from build123d import *

# Parameters (mm, degrees)
SKETCH1_W           = 16.5
SKETCH1_H           = 15.5
SKETCH1_W_2         = 12.5
SKETCH1_H_2         = 11.742424242
BOSS_EXTRUDE1_DEPTH = 5
BOSS_EXTRUDE2_DEPTH = 10
CUT_SWEEP1_START    = -6
CUT_SWEEP1_DEPTH    = 12


# Read off the part's stored shape, not the designer's step: Cut-Sweep1
with BuildPart() as part:
    # Sketch1 → Boss-Extrude1 (new body)
    with BuildSketch(Plane.XY):
        Rectangle(SKETCH1_W, SKETCH1_H)
        Rectangle(SKETCH1_W_2, SKETCH1_H_2, mode=Mode.SUBTRACT)
    extrude(amount=BOSS_EXTRUDE1_DEPTH)

    # Sketch3 → Boss-Extrude2 (add, symmetric)
    with BuildSketch(Plane(origin=(0, 0, 0), x_dir=(0, 0, -1), z_dir=(1, 0, 0))):
        with BuildLine():
            Line((13.022755533, 1.177389365), (0, -9.75))
            Line((0, -9.75), (0, 9.75))
            ThreePointArc((0, 9.75), (7.794535943, 7.412955642), (13.022755533, 1.177389365))
        make_face()
    extrude(amount=BOSS_EXTRUDE2_DEPTH, both=True)

    # Cut-Sweep1 outline → Cut-Sweep1 (cut)
    with BuildSketch(Plane.YZ.offset(CUT_SWEEP1_START)):
        Polygon((-3.793172037, -7.099071125), (4.667171481, 0), (-4.667171481, 0), (-7.649897695, -2.502804467), align=None)
    extrude(amount=CUT_SWEEP1_DEPTH, mode=Mode.SUBTRACT)


solid = part.part
Geometry: final body of the model. Coordinates: model frame, mm. A direction names the side the tool comes from. Give positions to 0.01 mm unless a question says otherwise; leave off trailing zeros. Write each loop counter-clockwise with the first axis right and the second up, starting at its lowest first coordinate (ties: lowest second). Pieces come first, ordered by that corner, then holes. Notation, with made-up numbers: M -40,6 L -23,6 A5 ccw -23,10 Z; hole C -8.75,-31 d1. An arc over 180 degrees is marked long. Answer in a Markdown table with one row per item. Add a question column.
(1) Section A-A on z = 0.5. Return loops of the section in (x, y), and give its area (3 significant figures).
(2) Section D-D on y = -7.25. Return loops of the section in (x, z), and give its area (3 significant figures).
(3) Ray query, line 1 (X direction, y = -3.5, z = 1.75); line 2 (X direction, y = -1.5, z = -1); line 3 (Y direction, x = -7.25, z = 1.75). Return the intervals inside material, ascending.
(4) Section C-C on x = -7.25. Return loops of the section in (y, z), and give its area (3 significant figures).
(5) First-contact query: pin 1 (2.5 mm diameter, centred on y = -2, z = 2, fed in from +X); pin 2 (1 mm diameter, centred on x = 6.5, z = -4.5, fed in from +Y); pin 3 (10 mm diameter, centred on x = 4, z = -4, fed in from +Y); pin 4 (2.5 mm diameter, centred on x = 1.5, z = 2.5, fed in from -Y). Flat tips, straight axial feed; report the tip coordinate or a pass-through.
(6) Mould query, pull axis Y, two halves, no side actions, for faces 6 (the flat face through (0, -5.871, 2)), 7 (the flat face through (0, -7, 5)), 8 (the flat face through (0, -7.75, 2)). Classes: +Y half, -Y half, draft (parallel to the pull), parting line (faces both ways), or undercut.
(7) Reachability of faces 1 (the flat face through (-0.1, -6.1, -1.2)), 2 (the flat face through (1, -5, 0)), 3 (the flat face through (-8.25, 0, 2)), 4 (the flat face through (0, 7.75, 2)), 5 (the flat face through (-6, -2, -3)) from +Z, -Z, +X, -X, +Y, -Y: full face, straight path, thin tool, end or side. Return the list, or none.
(8) Section B-B on x = 0.75. Return loops of the section in (y, z).
Result set:
| question | item | result |
|---|---|---|
| 1 | outline | M -8.25,-7.75 L 8.25,-7.75 L 8.25,7.75 L -8.25,7.75 Z; hole M -6.25,-5.87 L 6.25,-5.87 L 6.25,5.87 L -6.25,5.87 Z |
| 1 | area | 109 mm^2 |
| 2 | outline | M -10,-2.98 L -6,-2.98 L -6,-2.17 L 6,-2.17 L 6,-2.98 L 10,-2.98 L 10,0 L 8.25,0 L 8.25,5 L -8.25,5 L -8.25,0 L -10,0 Z |
| 2 | area | 132 mm^2 |
| 3 | line 1 | x = -8.25 to -6.25, 6.25 to 8.25 |
| 3 | line 2 | x = -10 to -6, 6 to 10 |
| 3 | line 3 | y = -7.75 to 7.75 |
| 4 | outline | M -9.75,0 L 1.18,-13.02 A14.19 ccw 9.75,0 L 7.75,0 L 7.75,5 L -7.75,5 L -7.75,0 Z |
| 4 | area | 229 mm^2 |
| 5 | pin 1 | stops at x = 8.25 |
| 5 | pin 2 | stops at y = 9.17 |
| 5 | pin 3 | stops at y = 9.75 |
| 5 | pin 4 | stops at y = -7.75 |
| 6 | face 6 | undercut |
| 6 | face 7 | draft |
| 6 | face 8 | -Y half |
| 7 | face 1 | -Z |
| 7 | face 2 | +Z |
| 7 | face 3 | +Z, -X, +Y, -Y |
| 7 | face 4 | +Z, +X, -X, +Y |
| 7 | face 5 | none |
| 8 | outline | M -9.75,0 L -7.65,-2.5 L -4.67,0 L -5.87,0 L -5.87,5 L -7.75,5 L -7.75,0 Z; M -3.79,-7.1 L 1.18,-13.02 A14.19 ccw 9.75,0 L 7.75,0 L 7.75,5 L 5.87,5 L 5.87,0 L 4.67,0 Z |
